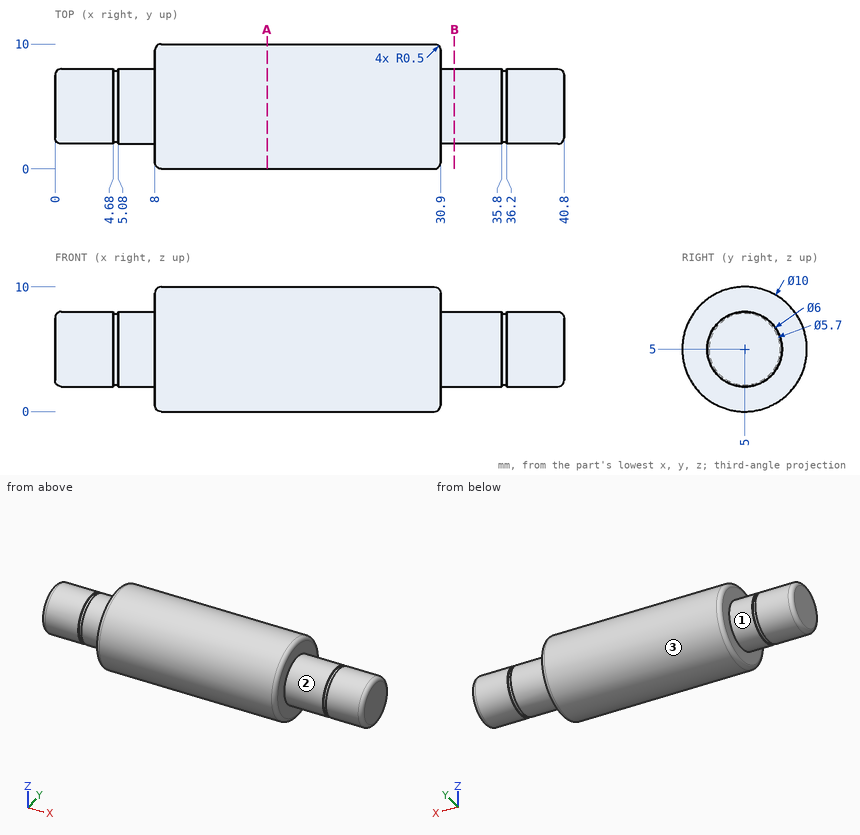
Answer from the drawing. Dimensions are ordinates in mm from the lowest x, y and z of the part. A direction names the side the tool comes from. Coordinates: 2 decimals unless noted, no trailing zeros. Write each loop counter-clockwise with the first axis right and the second up, starting at its lowest first coordinate (ties: lowest second). Pieces come first, ordered by that corner, then holes. Notation, with made-up numbers: (-11, 15) - (-1, 15) arc R8 cw to (-1, 30) - close; hole circle Ø1 at (82, 4.25). An arc over 180 degrees is marked (long way). Return JSON: item names as keys, results as strings.
1. The part is cut by section A-A on x = 17. Determine the outline of the cut face in (y, z), then the cut area to 3 significant figures.
Final values:
{"outline": "circle Ø10 at (5, 5)", "area": "78.5 mm^2"}
2. Which of the six approach directions +Z, -Z, +X, -X, +Y, -Y give full straight-line access (tool end or side, diameter ignored) to the marked faces 1, 2 and 3?
Final values:
{"face 1": "-X", "face 2": "+X", "face 3": "+X, -X"}
3. Consider line 1 along X through (y, z) = (9.25, 4.5); line 2 along Y through (x, z) = (11, 4.75); line 3 along Z through (x, y) = (37, 5). Determine where each line is inside the solid, lowest interval first.
Final values:
{"line 1": "8 to 30.9", "line 2": "0.01 to 9.99", "line 3": "2 to 8"}
4. The part is cut by section B-B on x = 32. Determine the outline of the cut face in (y, z).
Final values:
{"outline": "circle Ø6 at (5, 5)"}
5. Each of these flat-tipped pins is pushed along its axis until it touches: pin 1 Ø1 at (x, y) = (6, 5.5) entering from +Z; pin 2 Ø1.5 at (x, y) = (9, 4) entering from -Z. Where does it stop, or does it pass through?
Final values:
{"pin 1": "z = 8", "pin 2": "z = 0.01"}
